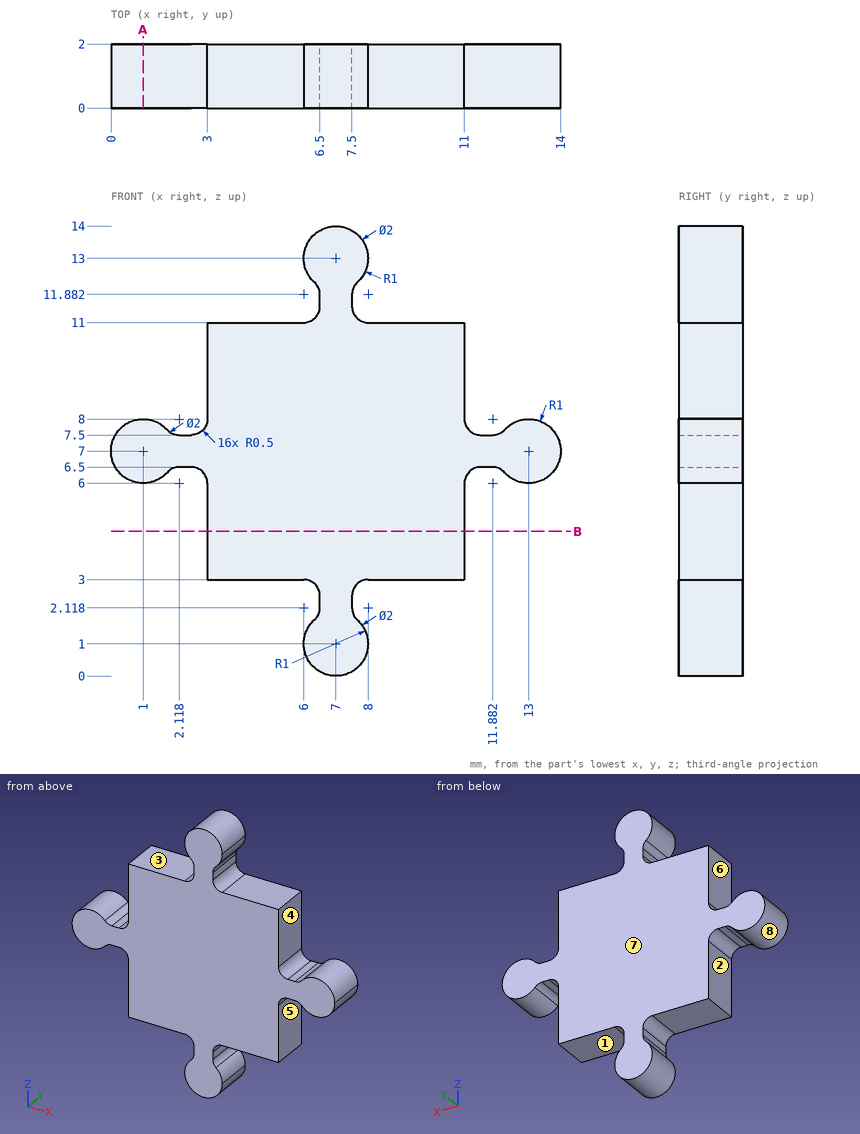
The figure shows three views and two pictorial views of one solid part (mm, origin at its lowest corner). Answer the questions. A direction names the side the tool comes from. Coordinates: 2 decimals unless noted, no trailing zeros. Loops run counter-clockwise (first coordinate to the right, second up) from the corner with the lowest first, then second, coordinate; pieces in that order, holes last.
1) Find section A-A on x = 1. Write down the section's boundary in (y, z), then the cut area to 3 significant figures.
2) Determine the mould class of the marked faces 5, 6, 7 and 8 for opening direction X: pulls with the +X half, pulls with the -X half, needs draft (parallel to the pull), parting line crosses it, or undercut.
3) A tool of negligible diameter and unlimited length cuts with its end or side. For the marked faces 1, 2, 3 and 4, from which of +Z, -Z, +X, -X, +Y, -Y can it reach the whole face along a straight path? Write none if from no direction.
4) Find the intervals of material crossed by L1, parallel to X at y = 0.4, z = 6.25; L2, parallel to Z at x = 5.5, y = 0.95, in increasing order.
5) Find section B-B on z = 4.5. Write down the section's boundary in (x, y), then the cut area to 3 significant figures.
6) Flat-ended cylindrical pins translate along their axes: pin 1 Ø1 at (x, y) = (9.5, 1) entering from +Z; pin 2 Ø0.6 at (x, y) = (5, 1) entering from -Z. Find the tip coordinate at first contact, or state that the pin passes through.
Values:
1. outline: (0, 6) - (2, 6) - (2, 8) - (0, 8) - close
1. area: 4.00 mm2
2. face 5: pulls with the +X half
2. face 6: pulls with the -X half
2. face 7: needs draft
2. face 8: undercut
3. face 1: -Z, +X, +Y, -Y
3. face 2: -Z, -X, +Y, -Y
3. face 3: +Z, -X, +Y, -Y
3. face 4: +Z, +X, +Y, -Y
4. L1: x = 0.34 to 1.66, 2.93 to 11.07, 12.34 to 13.66
4. L2: z = 3 to 11
5. outline: (3, 0) - (11, 0) - (11, 2) - (3, 2) - close
5. area: 16.0 mm2
6. pin 1: stops at z = 11
6. pin 2: stops at z = 3
